Autodesk Inventor part; units mm, degrees
ref_plane "YZ Plane" through (0, 0, 0) normal (1, 0, 0) x (0, 1, 0)
ref_plane "XZ Plane" through (0, 0, 0) normal (0, 1, 0) x (-1, 0, 0)
ref_plane "XY Plane" through (0, 0, 0) normal (0, 0, 1) x (1, 0, 0)
sketch "Sketch1" plane through (0, 0, 0) normal (1, 0, 0) x (0, 1, 0)
  line L0 (0, 49.99) -> (2, 49.99) construction
  line L1 (2, 49.99) -> (2, -49.99) construction
  line L2 (2, -49.99) -> (0, -49.99) construction
  line L3 (0, 49.99) -> (0, 0) construction
  line L4 (0, 0) -> (0, -49.99) construction
  arc A0 (46.99, 5) -> (2, 49.99) centre (2, 5) ccw construction
  arc A1 (2, -49.99) -> (46.99, -5) centre (2, -5) ccw construction
  line L5 (46.99, 5) -> (46.99, -5) construction
  arc A2 (2, -47.99) -> (44.99, -5) centre (2, -5) ccw construction
  line L6 (44.99, -5) -> (44.99, 5) construction
  arc A3 (44.99, 5) -> (2, 47.99) centre (2, 5) ccw construction
  line L7 (44.99, 5) -> (44.99, 49.99) construction
  dimension "d0" = 99.98
  dimension "d1" = 2
  dimension "d2" = 10
  dimension "d3" = 2
  dimension "d4" = 2
sketch "Sketch2" plane through (0, 0, 0) normal (1, 0, 0) x (0, 1, 0)
  line L0 (0, 49.99) -> (2, 49.99) construction
  line L1 (2, 49.99) -> (2, -49.99) construction
  line L2 (2, -49.99) -> (0, -49.99) construction
  line L3 (0, 49.99) -> (0, 0) construction
  line L4 (0, 0) -> (0, -49.99) construction
  arc A0 (46.99, 5) -> (2, 49.99) centre (2, 5) ccw construction
  arc A1 (2, -49.99) -> (46.99, -5) centre (2, -5) ccw construction
  line L5 (46.99, 5) -> (46.99, -5) construction
  arc A2 (2, -47.99) -> (44.99, -5) centre (2, -5) ccw construction
  line L6 (44.99, -5) -> (44.99, 5) construction
  arc A3 (44.99, 5) -> (2, 47.99) centre (2, 5) ccw construction
  line L7 (44.99, 5) -> (44.99, 49.99) construction
  line L8 (2, 49.99) -> (2, -47.99)
  arc A4 (2, -47.99) -> (44.99, -5) centre (2, -5) ccw
  line L9 (44.99, -5) -> (44.99, 18.265)
  arc A5 (44.99, 18.265) -> (2, 49.99) centre (2, 5) ccw
extrude "Extrusion1" add sketch "Sketch2" along normal blind 1.98
sketch "Sketch3" plane through (0, 0, 0) normal (-1, 0, 0) x (0, 0, 1)
  line L0 (26.265, 33.495) -> (26.265, 13.495)
  arc A0 (26.265, 13.495) -> (26.265, 33.495) centre (26.265, 23.495) ccw
  line L1 (-5, 44.99) -> (18.265, 44.99)
  line L2 (18.265, 44.99) -> (18.265, 23.495)
  line L3 (18.265, 23.495) -> (18.265, 2)
  line L4 (49.99, 2) -> (-47.99, 2)
  point P0 (0, 0)
  dimension "d7" = 20
  dimension "d8" = 8
extrude "Extrusion2" cut sketch "Sketch3" against normal blind 1
fillet "Fillet1" radius 2 1 edges at (0, 23.495, 36.265)
properties part number "BuddyRobotBaseDoor"
Can you work these out from the model? Positions are in its coordinate system, mm. Coordinates: 2 decimals unless noted, no trailing zeros. Write each loop counter-clockwise with the first axis right and the second up, starting at its lowest first coordinate (ties: lowest second). Pieces come first, ordered by that corner, then holes. Notation, with made-up numbers: (0.5, -30) -> (28.5, -30) arc R14 cw to (28.5, -25) -> close; hole circle Ø7 at (-21.75, 59.25). An arc over 180 degrees is marked (long way). Write each question's results on one line, items separated by ' | '. Start each with the question number.
Item 1: I'm going to push a flat-ended pin straight in: P1, Ø0.5, axis at x = 0.5, y = 27, coming from the +Z side. Where does the tip first touch, or does it pass through?
Item 2: If we section it at B-B, the plane z = -34.5: Write out the boundary of the cut face in (x, y).
Item 3: Please list where these lines run through material, in increasing order: probe 1 along Z at (x, y) = (0.6, 15.5) (3 decimals); probe 2 along X at (y, z) = (25.5, 35.5); probe 3 along Y at (x, z) = (0.15, -10.5).
Item 4: If we section it at A-A, the plane x = 1.35: Write out the boundary of the cut face in (y, z) (3 decimals), and give its area (3 significant figures).
Item 5: Thinking about a two-plate mould opening in Z: for faces 1 (the cylindrical face through (0.976, 28.391, 41.436)), 2 (the flat face through (1.98, 18, 2)), 3 (the flat face through (1, 24, 30)), 4 (the cylindrical face through (0.976, 32.731, -35.062)), which applies, released by +Z, released by -Z, zero draft, split by the parting line, or undercut?
Answer block:
1) P1: z = 42.57
2) outline: (0, 2) -> (1.98, 2) -> (1.98, 33.27) -> (0, 33.27) -> close
3) probe 1: -45.815 to 26.265, 32.765 to 47.917 | probe 2: 1 to 1.98 | probe 3: 2 to 44.64
4) outline: (2, -47.99) arc R42.99 ccw to (44.99, -5) -> (44.99, 18.265) arc R44.99 ccw to (2, 49.99) -> close | area: 3,450 mm²
5) face 1: released by +Z | face 2: zero draft | face 3: undercut | face 4: released by -Z
